Can you work these out from the model? Positions are in its coordinate system, mm. A direction names the side the tool comes from. Give positions to 0.01 mm unless a question says otherwise; leave off trailing zeros. Write each loop counter-clockwise with the first axis right and the second up, starting at its lowest first coordinate (ties: lowest second). Pieces come first, ordered by that corner, then holes.
1. Suppose I cut it at D-D (y = -10). Please give me the cut outline in (x, z) (1 decimal).
2. Suppose I cut it at A-A (z = 15.25). Please give me the cut outline in (x, y) (3 decimals), and give its area (3 significant figures).
3. If I drill on probe 1 along X at (y, z) = (-76.5, 13) (3 decimals); probe 2 along Z at (x, y) = (-3, -11.5); probe 3 along Z at (x, y) = (-10.5, -12) (3 decimals), over which ranges is the centre line in solid material (lowest first)?
4. Suppose I cut it at C-C (x = 2). Please give me the cut outline in (y, z) (1 decimal), and give its area (3 significant figures).
5. Suppose I cut it at B-B (y = -35.5). Please give me the cut outline in (x, z) (1 decimal), and give its area (3 significant figures).
6. Thinking about a two-plate mould opening in X: for faces 1 (the flat face through (24, -38.6, 4.7)), 2 (the flat face through (-28.575, -81, 9)), 3 (the flat face through (0, -10, 4.762)), 4 (the flat face through (-33.404, -87.419, 12.315)), which applies, pulls with the +X half, pulls with the -X half, needs draft (parallel to the pull), parting line crosses it, or undercut?
7. I'm going to push flat-ended pins straight in: pin 1 (2.5 mm diameter, centred on x = 1, z = 2, fed in from -Y); pin 2 (2.5 mm diameter, centred on x = -31.5, z = 21.5, fed in from +Y); pin 3 (12 mm diameter, centred on y = -68, z = 12, fed in from -X); pin 4 (10 mm diameter, centred on x = 29, z = 10, fed in from -Y). Where does each tip first touch, or does it pass through?
8. On a 3-axis mill with a long thin cutter (end or side, diameter ignored), from which of +Z, -Z, +X, -X, +Y, -Y can I reach the whole of each face in a straight line? I mean faces 5 (the flat face through (-4.762, -13, 6)), 6 (the flat face through (-33, -76.2, 14)), 7 (the flat face through (-17.618, -46.982, 4.696)), 8 (the flat face through (-33, -73.66, 22)), 9 (the flat face through (33.36, -83.187, 20.147)). Say none if no direction works.
```python
from build123d import *

# Parameters (mm, degrees)
F1_DEPTH = 9.525
F3_DEPTH = 9.525
F4_W     = 9.525
F4_H     = 9.525
F5_DEPTH = 4.7625
F6_W     = 9.525
F6_H     = 4.7625
F7_DEPTH = 4.7635
F8_SIZE  = 3.175


# Not quite as in the source:
# - a pattern or mirror of a feature is missing from the dataset's text; its kind, count and spacing are read off the source's solid


with BuildPart() as f1:
    # F0 (on Top) → F1 (new body)
    with BuildSketch(Plane.XY):
        Polygon((9.525, 0), (0, 0), (-9.525, 0), (-38.1, -76.2), (-38.1, -85.725), (-28.575, -85.725), (-28.575, -76.2), (-6.35, -16.9333333333), (0, -16.9333333333), (6.35, -16.9333333333), (28.575, -76.2), (28.575, -85.725), (38.1, -85.725), (38.1, -76.2), align=None)
    extrude(amount=F1_DEPTH)

    # F2 (on face) → F3 (join)
    with BuildSketch(Plane.YZ.offset(38.1)):
        Polygon((-85.725, 9.525), (-76.2, 9.525), (-76.2, 17.907), (-76.2, 20.447), (-73.66, 20.447), (-73.66, 23.622), (-79.6925, 23.622), (-86.7808208308, 16.5735), (-87.8366416617, 9.525), (-85.725, 0), align=None)
        Polygon((-76.2, 20.447), (-76.2, 17.907), (-73.66, 20.447), align=None)
    f3 = extrude(amount=-F3_DEPTH)

    # F3_copies: F3 across plane
    add(f3.mirror(Plane(origin=(0, 0, 0), x_dir=(0, 0, -1), z_dir=(-1, 0, 0))))

    # F4 (on face) → F5 (cut)
    with BuildSketch(Plane.XY.offset(9.525)):
        with Locations((0, -12.1708333333)):
            Rectangle(F4_W, F4_H)
    extrude(amount=-F5_DEPTH, mode=Mode.SUBTRACT)

    # F6 (on face) → F7 (cut, through all)
    with BuildSketch(Plane.XY.offset(4.7625)):
        with Locations((0, -14.5520833333)):
            Rectangle(F6_W, F6_H)
    extrude(amount=-F7_DEPTH, mode=Mode.SUBTRACT)

    # F8
    f8_edges = [f1.edges().sort_by_distance(p)[0] for p in [
        (38.1, -83.23666, 20.09775),
        (28.575, -83.23666, 20.09775),
        (-38.1, -83.23666, 20.09775),
        (-28.575, -83.23666, 20.09775),
    ]]
    chamfer(f8_edges, length=F8_SIZE)


solid = f1.part
```
Checks:
1. outline: (-13.3, 0) - (13.3, 0) - (13.3, 9.5) - (4.8, 9.5) - (4.8, 4.8) - (-4.8, 4.8) - (-4.8, 9.5) - (-13.3, 9.5) - close
2. outline: (-38.1, -83.609) - (-35.724, -86.979) - (-30.951, -86.979) - (-28.575, -83.609) - (-28.575, -76.2) - (-38.1, -76.2) - close; (28.575, -83.609) - (30.951, -86.979) - (35.724, -86.979) - (38.1, -83.609) - (38.1, -76.2) - (28.575, -76.2) - close
2. area: 189 mm2
3. probe 1: x = -38.1 to -28.575, 28.575 to 38.1
3. probe 2: z = 0 to 4.76
3. probe 3: z = 0 to 9.525
4. outline: (-12.2, 0) - (0, 0) - (0, 9.5) - (-7.4, 9.5) - (-7.4, 4.8) - (-12.2, 4.8) - close
4. area: 93.2 mm2
5. outline: (-22.8, 0) - (-13.3, 0) - (-13.3, 9.5) - (-22.8, 9.5) - close; (13.3, 0) - (22.8, 0) - (22.8, 9.5) - (13.3, 9.5) - close
5. area: 181 mm2
6. face 1: pulls with the +X half
6. face 2: undercut
6. face 3: undercut
6. face 4: needs draft
7. pin 1: stops at y = -12.17
7. pin 2: stops at y = -73.66
7. pin 3: stops at x = -37.07
7. pin 4: stops at y = -87.84
8. face 5: +Z, -Y
8. face 6: +X, -X, +Y
8. face 7: +Z, -Z, -Y
8. face 8: +Z, +X, -X, +Y
8. face 9: +Z, +X, -X, -Y
